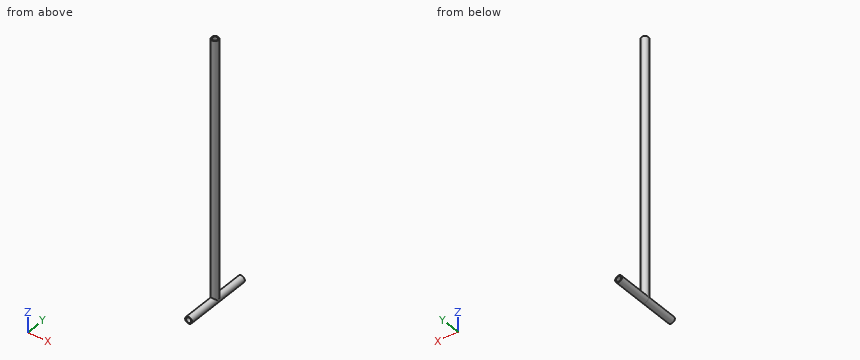
```python
from build123d import *

# Parameters (mm, degrees)
SKETCH3_R                = 4
SKETCH3_R_2              = 3
BOSS_EXTRUDE1_DEPTH      = 300
SKETCH6_R                = 4
SKETCH6_R_2              = 3
BOSS_EXTRUDE3_DEPTH      = 40
BOSS_EXTRUDE3_DEPTH_BACK = 40
SKETCH7_R                = 3
CUT_EXTRUDE1_DEPTH       = 1.0000001
CUT_EXTRUDE1_DEPTH_BACK  = 81.0000001


with BuildPart() as part:
    # Sketch3 → Boss-Extrude1 (new body)
    with BuildSketch(Plane.XY):
        Circle(SKETCH3_R)
        Circle(SKETCH3_R_2, mode=Mode.SUBTRACT)
    extrude(amount=BOSS_EXTRUDE1_DEPTH)

    # Sketch6 → Boss-Extrude3 (add, two sides)
    with BuildSketch(Plane(origin=(0, 0, 0), x_dir=(1, 0, 0), z_dir=(0, 1, 0))) as boss_extrude3_sk:
        Circle(SKETCH6_R)
        Circle(SKETCH6_R_2, mode=Mode.SUBTRACT)
    extrude(amount=BOSS_EXTRUDE3_DEPTH)
    extrude(boss_extrude3_sk.sketch, amount=-BOSS_EXTRUDE3_DEPTH_BACK)

    # Sketch7 → Cut-Extrude1 (cut, two sides)
    with BuildSketch(Plane.XZ.offset(40)) as cut_extrude1_sk:
        Circle(SKETCH7_R)
    extrude(amount=CUT_EXTRUDE1_DEPTH, mode=Mode.SUBTRACT)
    extrude(cut_extrude1_sk.sketch, amount=-CUT_EXTRUDE1_DEPTH_BACK, mode=Mode.SUBTRACT)


solid = part.part
```
Geometry check sheet. Reference: the model listing, model coordinates, mm. Round coordinates to 2 decimals unless told otherwise and drop trailing zeros. Order: outer loops, then holes, each group sorted by start corner. A loop starts at its lowest first (then second) coordinate and runs counter-clockwise, first axis right, second up. Notation, with made-up numbers: (-35.75, -33) - (-14.75, -33) arc R11 ccw to (-14.75, -25) - close; hole circle Ø2 at (1, 87). An arc over 180 degrees is marked (long way). Use a Markdown table: item, result. Add a question column.
1) Thickness scan on line 1 along X through (y, z) = (0, 229); line 2 along Y through (x, z) = (0.25, 280). Record the ranges inside material, lowest first.
2) Gauge pin test, flat ends, axial feed: P1, Ø2, axis at x = 2, y = -10.5, coming from the +Z side; P2, Ø4, axis at x = 0, z = 42, coming from the +Y side; P3, Ø1.5, axis at x = 1.5, z = 98.5, coming from the +Y side. Record the tip position at first contact, or that the pin passes through.
3) Section check A-A (x = 0). Record the cut outline in (y, z), then the cut area to 3 significant figures.
4) Section check B-B (y = -20.5). Record the cut outline in (x, z).
Established:
| question | item | result |
|---|---|---|
| 1 | line 1 | -4 to -3, 3 to 4 |
| 1 | line 2 | -3.99 to -2.99, 2.99 to 3.99 |
| 2 | P1 | z = 3.87 |
| 2 | P2 | y = 4 |
| 2 | P3 | y = 3.93 |
| 3 | outline | (-40, -4) - (40, -4) - (40, -3) - (-40, -3) - close; (-40, 3) - (40, 3) - (40, 4) - (4, 4) - (4, 300) - (3, 300) - (3, 4) - (-3, 4) - (-3, 300) - (-4, 300) - (-4, 4) - (-40, 4) - close |
| 3 | area | 752 mm2 |
| 4 | outline | circle Ø8 at (0, 0); hole circle Ø6 at (0, 0) |
